from build123d import *

# Parameters (mm, degrees)
F0_W     = 75
F0_H     = 50
F1_DEPTH = 65
F2_R     = 5
F3_R     = 12.5
F4_DEPTH = 50.001
F6_DEPTH = 75.001


with BuildPart() as f1:
    # F0 (on Front) → F1 (new body)
    with BuildSketch(Plane.XZ):
        with Locations((-0.09526, -25)):
            Rectangle(F0_W, F0_H)
    extrude(amount=F1_DEPTH)

    # F2
    f2_edges = [f1.edges().sort_by_distance(p)[0] for p in [
        (-0.09526, -65, 0),
        (-37.59526, -32.5, 0),
        (-0.09526, 0, 0),
        (37.40474, -32.5, 0),
    ]]
    fillet(f2_edges, radius=F2_R)

    # F3 (on face) → F4 (cut, through all)
    with BuildSketch(Plane.XY):
        with Locations((-2.59526, -35)):
            Circle(F3_R)
    extrude(amount=-F4_DEPTH, mode=Mode.SUBTRACT)

    # F5 (on face) → F6 (cut, through all)
    with BuildSketch(Plane(origin=(-37.59526, 0, 0), x_dir=(0, -1, 0), z_dir=(-1, 0, 0))):
        Polygon((34.392635, -39.305133), (42.407697, -33.964212), (44.2986, -24.520106), (38.957679, -16.505044), (29.513573, -14.614141), (21.498511, -19.955062), (19.607608, -29.399168), (24.948529, -37.41423), align=None)
    extrude(amount=-F6_DEPTH, mode=Mode.SUBTRACT)


solid = f1.part
Could you check a few things on this model? Use its own coordinates, in mm. A direction names the side the tool comes from. Give positions to 0.01 mm unless a question says otherwise; leave off trailing zeros. Order: outer loops, then holes, each group sorted by start corner. A loop starts at its lowest first (then second) coordinate and runs counter-clockwise, first axis right, second up.
1. Which directions (+Z, -Z, +X, -X, +Y, -Y) give clear straight access to the entire face, cutting with the end or side of a thin tool? Please do faces 1 (the flat face through (-25.877, -34.302, -15.573)), 2 (the cylindrical face through (-5.31, -47.2, -24.65)).
Answers below:
face 1: +X, -X
face 2: +Z, -Z
2. Suppose I cut it at A-A (z = -19). Write out the boundary of the cut face in (x, y).
Answers below:
outline: (-37.6, -65) - (37.4, -65) - (37.4, -40.62) - (8.57, -40.62) arc R12.5 cw to (-13.76, -40.62) - (-37.6, -40.62) - close; (-37.6, -22.93) - (-5.85, -22.93) arc R12.5 cw to (0.66, -22.93) - (37.4, -22.93) - (37.4, 0) - (-37.6, 0) - close
3. Suppose I cut it at C-C (y = -46). Write out the boundary of the cut face in (x, z).
Answers below:
outline: (-37.6, -50) - (-8.53, -50) - (-8.53, 0) - (-32.6, 0) arc R5 ccw to (-37.6, -5) - close; (3.34, -50) - (37.4, -50) - (37.4, -5) arc R5 ccw to (32.4, 0) - (3.34, 0) - close
4. I need wall thicknesses on L1, parallel to X at y = -35, z = -9.5; L2, parallel to Z at x = -32.5, y = -26.5; L3, parallel to Y at x = -14, z = -23.5. Which ranges of each line are inside material? Lowest first, please.
Answers below:
L1: x = -37.6 to -15.1, 9.9 to 37.4
L2: z = -50 to -37.72, -16.62 to 0
L3: y = -65 to -43.62, -20.79 to 0
5. Suppose I cut it at D-D (y = -33.5). Write out the boundary of the cut face in (x, z).
Answers below:
outline: (-37.6, -50) - (-15, -50) - (-15, -39.13) - (-37.6, -39.13) - close; (-37.6, -15.41) - (-15, -15.41) - (-15, 0) - (-32.6, 0) arc R5 ccw to (-37.6, -5) - close; (9.81, -50) - (37.4, -50) - (37.4, -39.13) - (9.81, -39.13) - close; (9.81, -15.41) - (37.4, -15.41) - (37.4, -5) arc R5 ccw to (32.4, 0) - (9.81, 0) - close
6. Thinking about a two-plate mould opening in Y: for faces 3 (the flat face through (-1, -65, -27)), 4 (the flat face through (22.819, -34.302, -15.573)), 5 (the cylindrical face through (35.979, -32.955, -1.504)), 6 (the cylindrical face through (0, -2, -1)), which applies, +Y half, -Y half, draft (parallel to the pull), parting line (faces both ways), or undercut?
Answers below:
face 3: -Y half
face 4: undercut
face 5: draft
face 6: +Y half
7. Suppose I cut it at B-B (x = 17). Write out the boundary of the cut face in (y, z).
Answers below:
outline: (-65, -50) - (0, -50) - (0, -5) arc R5 ccw to (-5, 0) - (-60, 0) arc R5 ccw to (-65, -5) - close; hole (-44.3, -24.52) - (-42.41, -33.96) - (-34.39, -39.31) - (-24.95, -37.41) - (-19.61, -29.4) - (-21.5, -19.96) - (-29.51, -14.61) - (-38.96, -16.51) - close
